For this review, take the finished solid that the model builds, in its own axes (mm). Face numbers are marked on the shaded views. Give positions to 0.01 mm unless a question says otherwise; leave off trailing zeros. Loops run counter-clockwise (first coordinate to the right, second up) from the corner with the lowest first, then second, coordinate; pieces in that order, holes last.
Autodesk Inventor part; units mm, degrees
ref_plane "YZ Plane" through (0, 0, 0) normal (1, 0, 0) x (0, 1, 0)
ref_plane "XZ Plane" through (0, 0, 0) normal (0, 1, 0) x (-1, 0, 0)
ref_plane "XY Plane" through (0, 0, 0) normal (0, 0, 1) x (1, 0, 0)
sketch "Sketch1" plane through (0, 0, 0) normal (0, 0, 1) x (1, 0, 0)
  line L0 (0, 19.9009) -> (0, -19.9009)
  line L1 (33.5661, 19.9009) -> (33.5661, -19.9009)
  line L2 (33.5661, -19.9009) -> (0, -19.9009)
  line L3 (33.5661, 19.9009) -> (30.1625, 19.9009)
  line L4 (30.1625, 19.9009) -> (30.1625, -15.8369)
  line L5 (30.1625, -15.8369) -> (0, -15.8369)
  point P0 (0, 0)
  dimension "d0" = 39.8018
  dimension "d1" = 19.9009
  dimension "d2" = 39.8018
  dimension "d3" = 19.9009
  dimension "d4" = 67.1322
  dimension "d5" = 60.325
  dimension "d7" = 35.7378
revolve "Revolution1" add sketch "Sketch1" angle 360 about axis through (0, 19.9009, 0) along (0, -1, 0)
chamfer "Chamfer1" distance 1.5875 angle 45 2 edges at (-33.5661, 19.9009, 0) (-33.5661, -19.9009, 0)
equation "\"d0\" = d2"
properties part number "Flat Cap External 2 IN" material "PVC-Piping"
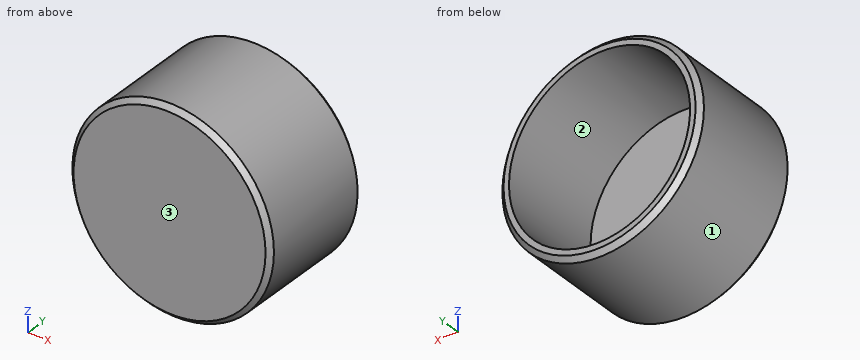
Item 1: Take a section at A-A on x = 0. Give the boundary of the cut face in (y, z).
Answer:
outline: (-19.9, -31.98) - (-18.31, -33.57) - (18.31, -33.57) - (19.9, -31.98) - (19.9, -30.16) - (-15.84, -30.16) - (-15.84, 30.16) - (19.9, 30.16) - (19.9, 31.98) - (18.31, 33.57) - (-18.31, 33.57) - (-19.9, 31.98) - close
Item 2: Take a section at B-B on z = 0. Give the boundary of the cut face in (x, y), and give its area (3 significant figures).
Answer:
outline: (-33.57, -18.31) - (-31.98, -19.9) - (31.98, -19.9) - (33.57, -18.31) - (33.57, 18.31) - (31.98, 19.9) - (30.16, 19.9) - (30.16, -15.84) - (-30.16, -15.84) - (-30.16, 19.9) - (-31.98, 19.9) - (-33.57, 18.31) - close
area: 511 mm2
Item 3: Take a section at C-C on y = -2.5. Give the boundary of the cut face in (x, z) (1 decimal).
Answer:
outline: circle Ø67.1 at (0, 0); hole circle Ø60.3 at (0, 0)
Item 4: For L1, parallel to Z at x = 0, y = 1; L2, parallel to Z at x = 1, y = -14; L3, parallel to Y at x = -24, z = 9, list the stretches that pass through material, from the lowest coordinate up.
Answer:
L1: z = -33.57 to -30.16, 30.16 to 33.57
L2: z = -33.55 to -30.15, 30.15 to 33.55
L3: y = -19.9 to -15.84
Item 5: Clearance check with flat-ended pins moving along their axes: pin 1 Ø3 at (x, z) = (-22, 12) entering from +Y; pin 2 Ø2 at (x, y) = (1, 13) entering from +Z; pin 3 Ø2 at (y, z) = (-8.5, 21) entering from -X; pin 4 Ø3 at (y, z) = (-5.5, -0.5) entering from +X. State where each tip first meets the part, or that it passes through.
Answer:
pin 1: stops at y = -15.84
pin 2: stops at z = 33.57
pin 3: stops at x = -26.96
pin 4: stops at x = 33.57
Item 6: The part is to be moulded in two halves that separate along X. For the marked faces 1, 2 and 3, say which applies: released by +X, released by -X, zero draft, split by the parting line, or undercut.
Answer:
face 1: split by the parting line
face 2: undercut
face 3: zero draft
